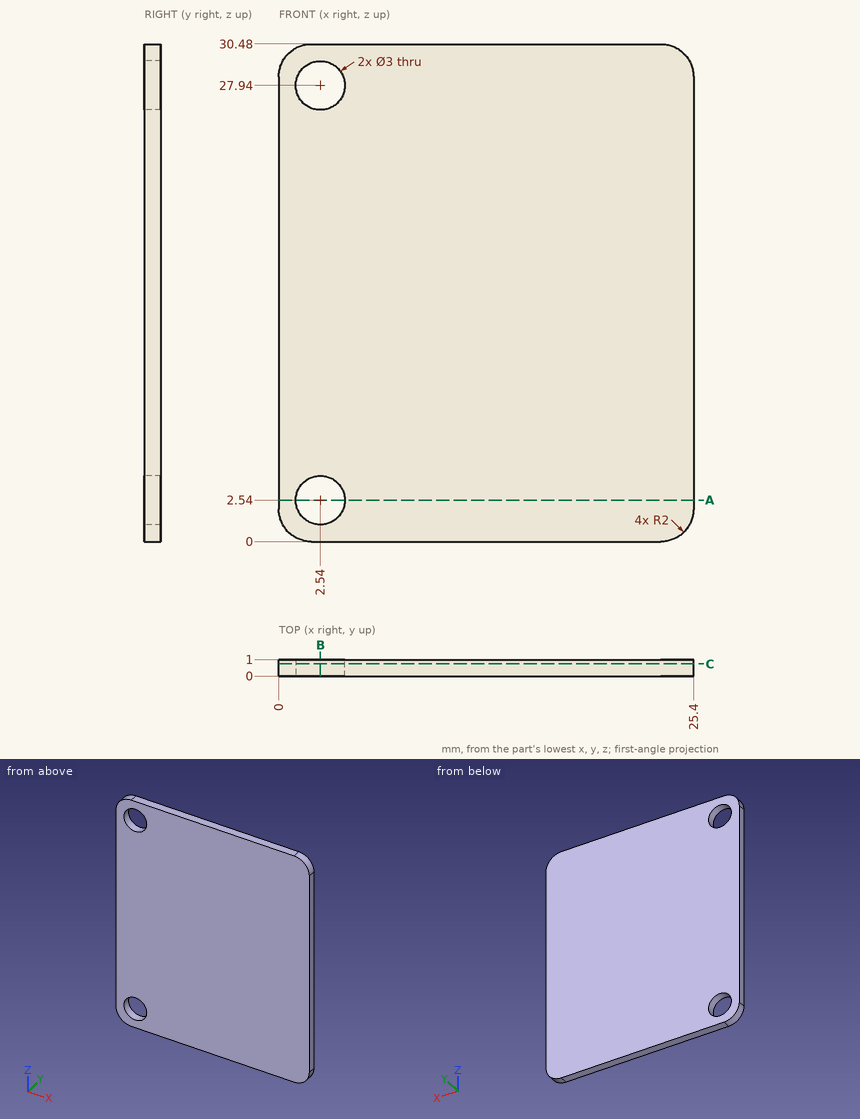
Geometry: see drawing. Coordinates: mm, zero at the bounding-box minimum. Coordinates: 2 decimals unless noted, no trailing zeros. Write each loop counter-clockwise with the first axis right and the second up, starting at its lowest first coordinate (ties: lowest second). Pieces come first, ordered by that corner, then holes.
1) Section B-B on x = 2.54. Output: boundary loops of the cut face in (y, z).
2) Section C-C on y = 0.75. Output: boundary loops of the cut face in (x, z), and give its area (3 significant figures).
3) Pin query (flat end, axial travel): pin 1 Ø2.5 at (x, z) = (2.54, 2.54) entering from -Y. Return the tip coordinate at first contact, or that it passes through.
4) Material intervals for line 1 along Z through (x, y) = (2.54, 0.75); line 2 along X through (y, z) = (0.2, 27.94); line 3 along X through (y, z) = (0.35, 3), sorted ascending.
5) Section A-A on z = 2.54. Output: boundary loops of the cut face in (x, y), and give its area (3 significant figures).
Check result:
1. outline: (0, 0) - (1, 0) - (1, 1.04) - (0, 1.04) - close; (0, 4.04) - (1, 4.04) - (1, 26.44) - (0, 26.44) - close; (0, 29.44) - (1, 29.44) - (1, 30.48) - (0, 30.48) - close
2. outline: (0, 2) arc R2 ccw to (2, 0) - (23.4, 0) arc R2 ccw to (25.4, 2) - (25.4, 28.48) arc R2 ccw to (23.4, 30.48) - (2, 30.48) arc R2 ccw to (0, 28.48) - close; hole circle Ø3 at (2.54, 2.54); hole circle Ø3 at (2.54, 27.94)
2. area: 757 mm2
3. pin 1: passes through
4. line 1: z = 0 to 1.04, 4.04 to 26.44, 29.44 to 30.48
4. line 2: x = 0 to 1.04, 4.04 to 25.4
4. line 3: x = 0 to 1.11, 3.97 to 25.4
5. outline: (0, 0) - (1.04, 0) - (1.04, 1) - (0, 1) - close; (4.04, 0) - (25.4, 0) - (25.4, 1) - (4.04, 1) - close
5. area: 22.4 mm2
